Here's how the part is built. I have some questions about the finished solid (model axes, mm). A direction names the side the tool comes from. Give positions to 0.01 mm unless a question says otherwise; leave off trailing zeros. Loops run counter-clockwise (first coordinate to the right, second up) from the corner with the lowest first, then second, coordinate; pieces in that order, holes last. Notation, with made-up numbers: (-16, 45.5) -> (36, 45.5) arc R23 ccw to (36, 55.5) -> close; hole circle Ø5 at (-3, 60). An arc over 180 degrees is marked (long way). Answer in a Markdown table with one row per item. Add a question column.
Item 1: If we section it at D-D (y = 0.65): Write out the boundary of the cut face in (x, z).
Item 2: If we section it at A-A (z = -40.5): Write out the boundary of the cut face in (x, y), then the cut area to 3 significant figures.
Item 3: Which directions (+Z, -Z, +X, -X, +Y, -Y) give clear straight access to the entire face, cutting with the end or side of a thin tool? Please do faces 1 (the face through (-120, 1, -25)), 2 (the face through (-110, 1, -25)).
Item 4: If we section it at C-C (x = -36.5): Write out the boundary of the cut face in (y, z), then the cut area to 3 significant figures.
Item 5: We'd pull the mould along Z, two halves only. Please class faces 3 (the face through (-36.13, 0.99, -38.84)), 4 (the face through (-59, 1, 0)), 5 (the face through (-61, 1, -50)), 6 (the face through (0, 1, -25)): released by +Z, released by -Z, zero draft, split by the parting line, or undercut.
Item 6: If I drill on line 1 (Z direction, x = -36.5, y = 1); line 2 (Z direction, x = -65, y = 1.6); line 3 (X direction, y = 1.2, z = -15.5), over which ranges is the centre line in solid material (lowest first)?
Item 7: If we section it at B-B (x = -15): Write out the boundary of the cut face in (y, z).
Item 8: For P1, Ø1, axis at x = -85, y = 1.5, coming from the +Z side, with a flat end and sliding along its axis, tell me the tip position at first contact or that it passes through.
Autodesk Inventor part; units mm, degrees
ref_plane "YZ Plane" through (0, 0, 0) normal (1, 0, 0) x (0, 1, 0)
ref_plane "XZ Plane" through (0, 0, 0) normal (0, 1, 0) x (-1, 0, 0)
ref_plane "XY Plane" through (0, 0, 0) normal (0, 0, 1) x (1, 0, 0)
sketch "Skizze1" plane through (0, 0, 0) normal (0, 1, 0) x (-1, 0, 0)
  line L0 (0, 0) -> (120, 0)
  line L1 (120, 0) -> (120, -50)
  line L2 (120, -50) -> (0, -50)
  line L3 (0, -50) -> (0, 0)
  line L4 (110, -37.5) -> (38, -37.5)
  line L5 (38, -37.5) -> (38, -12.5)
  line L6 (38, -12.5) -> (110, -12.5)
  line L7 (110, -12.5) -> (110, -37.5)
  line L8 (114, -43) -> (34, -43)
  line L9 (34, -43) -> (34, -7)
  line L10 (34, -7) -> (114, -7)
  line L11 (114, -7) -> (114, -43)
  circle A0 centre (111.5, -40.5) radius 1.7
  circle A1 centre (36.5, -40.5) radius 1.7
  circle A2 centre (111.5, -9.5) radius 1.7
  circle A3 centre (36.5, -9.5) radius 1.7
  circle A4 centre (15, -25) radius 3.5
  dimension "d0" = 120
  dimension "d1" = 50
  dimension "d2" = 72
  dimension "d3" = 25
  dimension "d4" = 80
  dimension "d5" = 36
  dimension "d6" = 5.5
  dimension "d7" = 5.5
  dimension "d8" = 4
  dimension "d9" = 4
  dimension "d10" = 3.4
  dimension "d11" = 3.4
  dimension "d12" = 75
  dimension "d13" = 2.5
  dimension "d14" = 2.5
  dimension "d15" = 3.4
  dimension "d16" = 3.4
  dimension "d17" = 2.5
  dimension "d18" = 2.5
  dimension "d19" = 31
  dimension "d20" = 2.5
  dimension "d21" = 2.5
  dimension "d22" = 2.5
  dimension "d23" = 7
  dimension "d24" = 7
  dimension "d25" = 15
  dimension "d26" = 6
extrude "Extrusion1" add sketch "Skizze1" along normal blind 2 contours L0 L1 L2 L3 | L8 L9 L10 L11
equation "\"d10\" = d15"
equation "\"d11\" = d15"
equation "\"d16\" = d15"
equation "\"Biegeradius\" = Stärke"
equation "\"BreiteBiegungsfreistellung\" = Stärke"
equation "\"TiefeBiegungsfreistellung\" = 0.5 * Stärke"
equation "\"GrößeEckenfreistellung\" = 4 * Stärke"
equation "\"MinimalRest\" = 2 * Stärke"
equation "\"Übergangsradius\" = Biegeradius"
equation "\"JacobiRadiusGröße\" = Biegeradius"
equation "\"Abstandsgröße\" = Stärke"
properties part number "Bedienfeld"
Recorded:
| question | item | result |
|---|---|---|
| 1 | outline | (-120, -50) -> (0, -50) -> (0, 0) -> (-120, 0) -> close; hole circle Ø3.4 at (-111.5, -40.5); hole circle Ø3.4 at (-111.5, -9.5); hole (-110, -37.5) -> (-38, -37.5) -> (-38, -12.5) -> (-110, -12.5) -> close; hole circle Ø3.4 at (-36.5, -40.5); hole circle Ø3.4 at (-36.5, -9.5); hole circle Ø7 at (-15, -25) |
| 2 | outline | (-120, 0) -> (-113.2, 0) -> (-113.2, 2) -> (-120, 2) -> close; (-109.8, 0) -> (-38.2, 0) -> (-38.2, 2) -> (-109.8, 2) -> close; (-34.8, 0) -> (0, 0) -> (0, 2) -> (-34.8, 2) -> close |
| 2 | area | 226 mm^2 |
| 3 | face 1 | +Z, -Z, -X, +Y, -Y |
| 3 | face 2 | +Y, -Y |
| 4 | outline | (0, -50) -> (2, -50) -> (2, -42.2) -> (0, -42.2) -> close; (0, -38.8) -> (2, -38.8) -> (2, -11.2) -> (0, -11.2) -> close; (0, -7.8) -> (2, -7.8) -> (2, 0) -> (0, 0) -> close |
| 4 | area | 86.4 mm^2 |
| 5 | face 3 | undercut |
| 5 | face 4 | released by +Z |
| 5 | face 5 | released by -Z |
| 5 | face 6 | zero draft |
| 6 | line 1 | z = -50 to -42.2, -38.8 to -11.2, -7.8 to 0 |
| 6 | line 2 | z = -50 to -37.5, -12.5 to 0 |
| 6 | line 3 | x = -120 to -110, -38 to 0 |
| 7 | outline | (0, -50) -> (2, -50) -> (2, -28.5) -> (0, -28.5) -> close; (0, -21.5) -> (2, -21.5) -> (2, 0) -> (0, 0) -> close |
| 8 | P1 | stops at z = 0 |
